from build123d import *

# Parameters (mm, degrees)
CONG_1_R                = 0.5
ENL_V_START             = -23
ESQUISSE9_R             = 3.9
ENL_V_MAT_EXTRU_4_DEPTH = 23
ESQUISSE10_W            = 39.610149942
ESQUISSE10_H            = 38.899653979
ENL_V_MAT_EXTRU_5_DEPTH = 43.652784254


with BuildPart() as part:
    # Esquisse1 → Base-Révolution (revolve)
    with BuildSketch(Plane.XY, mode=Mode.PRIVATE) as base_r_volution_sk:
        Polygon((0, 0), (0, 8.5), (1.4, 8.5), (1.4, 7.15), (9.9, 7.15), (9.9, 6), (19.9, 6), (19.9, 4.5), (26.9, 4.5), (28.9, 2.5), (28.9, 1.5), (32.4, 1.5), (32.4, 1.769872981), (34.9, 1.1), (34.9, 0), align=None)
    revolve(base_r_volution_sk.sketch.rotate(Axis((0, 0, 0), (1, 0, 0)), 90), axis=Axis((0, 0, 0), (1, 0, 0)))

    # Esquisse2 → Boss.-Révol.1 (revolve)
    with BuildSketch(Plane.XY):
        Polygon((8.6, 23), (8.6, -4), (12.5, -4), (12.5, -6.5), (6.1, -6.5), (6.1, 23), align=None)
    revolve(axis=Axis((12.5, 24, 0), (0, -1, 0)))

    # Esquisse7 → Enlèvement de matière-Révolution1 (revolve, cut)
    with BuildSketch(Plane.XY, mode=Mode.PRIVATE) as enl_vement_de_mati_re_r_volution1_sk:
        Polygon((34.9, 0.8), (34.9, 0), (0, 0), (0, 5.65), (8, 5.65), (8, 3.9), (18.5, 3.9), (18.5, 2), (26.5, 2), (26.5, 0.8), align=None)
    revolve(enl_vement_de_mati_re_r_volution1_sk.sketch.rotate(Axis((36, 0, 0), (-1, 0, 0)), 90), axis=Axis((36, 0, 0), (-1, 0, 0)), mode=Mode.SUBTRACT)

    # Congé1
    cong_1_edges = [part.edges().sort_by_distance(p)[0] for p in [
        (19.9, 0, -6),
        (9.9, -2.157400318, 6.816753177),
    ]]
    fillet(cong_1_edges, radius=CONG_1_R)

    # Esquisse9 → Enlèv. mat.-Extru.4 (cut)
    with BuildSketch(Plane(origin=(0, 23, 0), x_dir=(-1, 0, 0), z_dir=(0, 1, 0)).offset(ENL_V_START)):
        with Locations((-12.5, 0)):
            Circle(ESQUISSE9_R)
    extrude(amount=ENL_V_MAT_EXTRU_4_DEPTH, mode=Mode.SUBTRACT)

    # Esquisse10 → Enlèv. mat.-Extru.5 (cut, through all)
    with BuildSketch(Plane.XY):
        with Locations((16.621088043, 7.131584007)):
            Rectangle(ESQUISSE10_W, ESQUISSE10_H)
    extrude(amount=ENL_V_MAT_EXTRU_5_DEPTH, mode=Mode.SUBTRACT)


solid = part.part
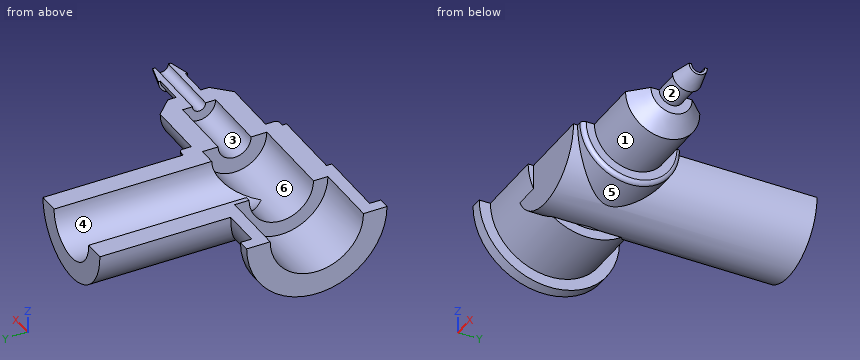
Can you work these out from the model? Positions are in its coordinate system, mm. Face numbers are marked on the shaded views. A direction names the side the tool comes from. Coordinates: 2 decimals unless noted, no trailing zeros. Write each loop counter-clockwise with the first axis right and the second up, starting at its lowest first coordinate (ties: lowest second). Pieces come first, ordered by that corner, then holes. Notation, with made-up numbers: (46, 33) - (70, 33) arc R17 ccw to (70, 58) - close; hole circle Ø10 at (-9, 38.25). An arc over 180 degrees is marked (long way). Return JSON: item names as keys, results as strings. Group by question number.
Item 1: If we section it at A-A (x = 12.5): Write out the boundary of the cut face in (y, z), then the cut area to 3 significant figures.
Item 2: We'd pull the mould along Y, two halves only. Please class the marked faces 4, 5 and 6: pulls with the +Y half, pulls with the -Y half, needs draft (parallel to the pull), parting line crosses it, or undercut.
Item 3: If we section it at C-C (x = 28): Write out the boundary of the cut face in (y, z), then the cut area to 3 significant figures.
Item 4: Which directions (+Z, -Z, +X, -X, +Y, -Y) give clear straight access to the entire face, cutting with the end or side of a thin tool? Please do the marked faces 1, 2 and 3.
Item 5: I'm going to push flat-ended pins straight in: pin 1 Ø3 at (x, z) = (29, -3.5) entering from +Y; pin 2 Ø0.6 at (y, z) = (1, -1.5) entering from -X; pin 3 Ø2 at (y, z) = (12, -3.5) entering from +X; pin 4 Ø1.5 at (x, z) = (23, -6.5) entering from -Y. Where does each tip first touch, or does it pass through?
Item 6: If we section it at B-B (y = 10.5): Write out the boundary of the cut face in (x, z).
Item 7: Please list where these lines run through material, in increasing order: probe 1 along Y at (x, z) = (10, -5.5); probe 2 along Z at (x, y) = (15.5, 8); probe 3 along X at (y, z) = (-2, -7.25).
Return value:
{
 "1": {"outline": "(-6.5, -6.4) - (23, -6.4) - (23, -3.9) - (0, -3.9) arc R3.9 cw to (-3.9, 0) - (-6.5, 0) - close", "area": "87.2 mm^2"},
 "2": {"face 4": "needs draft", "face 5": "parting line crosses it", "face 6": "undercut"},
 "3": {"outline": "(-3.4, 0) arc R3.4 ccw to (3.4, 0) - (0.8, 0) arc R0.8 cw to (-0.8, 0) - close", "area": "17.2 mm^2"},
 "4": {"face 1": "-Z, +X", "face 2": "-Z", "face 3": "+Z, -X"},
 "5": {"pin 1": "stops at y = 2.49", "pin 2": "stops at x = 18.5", "pin 3": "stops at x = 18.39", "pin 4": "passes through"},
 "6": {"outline": "(6.1, 0) arc R6.4 ccw to (18.9, 0) - (16.4, 0) arc R3.9 cw to (8.6, 0) - close"},
 "7": {"probe 1": "y = -6.5 to 23", "probe 2": "z = -5.65 to -2.49", "probe 3": "x = 0 to 1.4"}
}
